```python
from build123d import *

# Parameters (mm, degrees)
BOSS_EXTRUDE1_DEPTH             = 15
H_0_266_DIAMETER_HOLE1_D        = 6.7564
SKETCH5_W                       = 40
SKETCH5_H                       = 16
SKETCH5_W_2                     = 232
SKETCH5_H_2                     = 20.916111238
CUT_EXTRUDE1_DEPTH              = 243.332416321
SKETCH6_W                       = 237.036778435
SKETCH6_H                       = 127.431795429
CUT_EXTRUDE2_DEPTH              = 243.332416321
SKETCH10_W                      = 30
SKETCH10_H                      = 30
BOSS_EXTRUDE3_DEPTH             = 300
SKETCH11_R                      = 6.35
CUT_EXTRUDE4_DEPTH              = 400
SKETCH13_W                      = 600
SKETCH13_H                      = 44.158972604
BOSS_EXTRUDE4_DEPTH             = 3
SKETCH14_W                      = 268.104744415
SKETCH14_H                      = 124.61591485
CUT_EXTRUDE5_DEPTH              = 30
SKETCH15_W                      = 12.7
SKETCH15_H                      = 12.7
CUT_EXTRUDE6_DEPTH              = 385
BOSS_EXTRUDE5_REACH             = 353.137
SKETCH16_R                      = 3.3782
BOSS_EXTRUDE5_DIRECTION_2_REACH = 353.137
CHAMFER1_SIZE                   = 30


with BuildPart() as part:
    # Sketch1 → Boss-Extrude1 (new, symmetric)
    with BuildSketch(Plane.XY):
        with BuildLine():
            Line((-225, 15), (225, 15))
            ThreePointArc((225, 15), (240, 0), (225, -15))
            Line((225, -15), (-225, -15))
            ThreePointArc((-225, -15), (-240, 0), (-225, 15))
        make_face()
    extrude(amount=BOSS_EXTRUDE1_DEPTH, both=True)

    # H (0.266) Diameter Hole1 (through all)
    with Locations(Plane.XY.offset(15)):
        with Locations((-225, 0), (225, 0)):
            Hole(H_0_266_DIAMETER_HOLE1_D / 2)

    # Sketch5 → Cut-Extrude1 (cut, through all)
    with BuildSketch(Plane(origin=(0, 15, 0), x_dir=(1, 0, 0), z_dir=(0, 1, 0))):
        with Locations((-237, 0)):
            Rectangle(SKETCH5_W, SKETCH5_H)
        with Locations((141, 18.458055619)):
            Rectangle(SKETCH5_W_2, SKETCH5_H_2)
        with Locations((141, -18.458055619)):
            Rectangle(SKETCH5_W_2, SKETCH5_H_2)
    extrude(amount=-CUT_EXTRUDE1_DEPTH, mode=Mode.SUBTRACT)

    # Sketch6 → Cut-Extrude2 (cut, through all)
    with BuildSketch(Plane(origin=(0, 15, 0), x_dir=(1, 0, 0), z_dir=(0, 1, 0))):
        with Locations((-293.518389218, -4.674139215)):
            Rectangle(SKETCH6_W, SKETCH6_H)
    extrude(amount=-CUT_EXTRUDE2_DEPTH, mode=Mode.SUBTRACT)

    # Sketch10 → Boss-Extrude3 (add)
    with BuildSketch(Plane.ZY.offset(175)):
        Rectangle(SKETCH10_W, SKETCH10_H)
    extrude(amount=BOSS_EXTRUDE3_DEPTH)

    # Sketch11 → Cut-Extrude4 (cut)
    with BuildSketch(Plane.ZY.offset(475)):
        with Locations((0, 3)):
            Circle(SKETCH11_R)
    extrude(amount=-CUT_EXTRUDE4_DEPTH, mode=Mode.SUBTRACT)

    # Sketch13 → Boss-Extrude4 (add)
    with BuildSketch(Plane(origin=(0, -15, 0), x_dir=(-1, 0, 0), z_dir=(0, -1, 0))):
        with Locations((49.98, 0)):
            Rectangle(SKETCH13_W, SKETCH13_H)
    extrude(amount=BOSS_EXTRUDE4_DEPTH)

    # Sketch14 → Cut-Extrude5 (cut)
    with BuildSketch(Plane(origin=(0, 15, 0), x_dir=(1, 0, 0), z_dir=(0, 1, 0))):
        with Locations((-419.052372208, 3.913950599)):
            Rectangle(SKETCH14_W, SKETCH14_H)
    extrude(amount=-CUT_EXTRUDE5_DEPTH, mode=Mode.SUBTRACT)

    # Sketch15 → Cut-Extrude6 (cut)
    with BuildSketch(Plane.ZY.offset(285)):
        with Locations((0, 3)):
            Rectangle(SKETCH15_W, SKETCH15_H)
    extrude(amount=-CUT_EXTRUDE6_DEPTH, mode=Mode.SUBTRACT)

    # Boss-Extrude5: up to this face of the body (flat: up to its plane)
    boss_extrude5_end = Plane(part.part.faces().sort_by_distance((-130, 0, 15))[0])
    # Sketch16 → Boss-Extrude5 (add, up to the picked face)
    with BuildSketch(Plane.XY, mode=Mode.PRIVATE) as boss_extrude5_sk1:
        with Locations((225, 0)):
            Circle(SKETCH16_R)
    boss_extrude5_tool1 = split(extrude(boss_extrude5_sk1.sketch, amount=BOSS_EXTRUDE5_REACH, mode=Mode.PRIVATE), bisect_by=boss_extrude5_end, keep=Keep.BOTH, mode=Mode.PRIVATE)
    add(boss_extrude5_tool1.solids().sort_by(Axis((225, 0, 0), (0, 0, 1)))[0])

    # Boss-Extrude5 direction 2: up to this face of the body (flat: up to its plane)
    boss_extrude5_direction_2_end = Plane(part.part.faces().sort_by_distance((-130, 0, -15))[0])
    # Sketch16 → Boss-Extrude5 direction 2 (add, up to the picked face)
    with BuildSketch(Plane.XY, mode=Mode.PRIVATE) as boss_extrude5_direction_2_sk1:
        with Locations((225, 0)):
            Circle(SKETCH16_R)
    boss_extrude5_direction_2_tool1 = split(extrude(boss_extrude5_direction_2_sk1.sketch, amount=-BOSS_EXTRUDE5_DIRECTION_2_REACH, mode=Mode.PRIVATE), bisect_by=boss_extrude5_direction_2_end, keep=Keep.BOTH, mode=Mode.PRIVATE)
    add(boss_extrude5_direction_2_tool1.solids().sort_by(Axis((225, 0, 0), (0, 0, -1)))[0])

    # Chamfer1
    chamfer1_edges = [part.edges().sort_by_distance(p)[0] for p in [
        (25, 15, 11.5),
        (25, 15, -11.5),
    ]]
    chamfer(chamfer1_edges, length=CHAMFER1_SIZE - 0.0001)  # a hair under: the kernel refuses the full size


solid = part.part
```
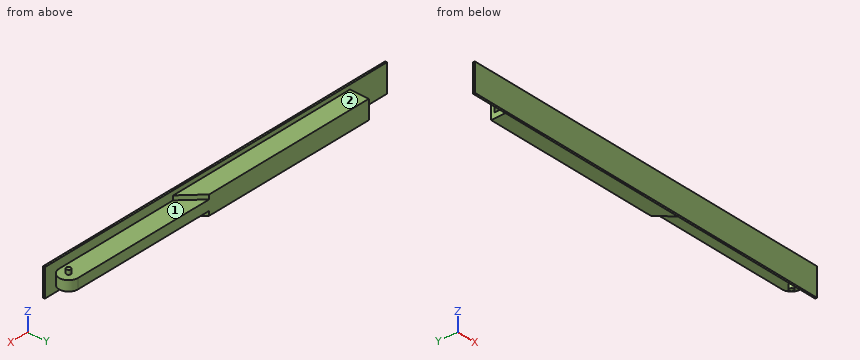
For this review, take the finished solid that the model builds, in its own axes (mm). Face numbers are marked on the shaded views. Coordinates: 2 decimals unless noted, no trailing zeros. Loops run counter-clockwise (first coordinate to the right, second up) from the corner with the lowest first, then second, coordinate; pieces in that order, holes last.
1. Insertion check: P1, Ø3, axis at x = -150, y = 3, coming from the -Z side; P2, Ø5, axis at y = -5.5, z = 2.5, coming from the +X side; P3, Ø3, axis at x = 130, y = 4, coming from the -Z side. Each pin has a flat end and moves straight along its axis. Give the tip position at first contact, or say it passes through.
2. Add section B-B, the plane x = 204. Give the boundary of the cut face in (y, z), then the cut area to 3 significant figures.
3. Mouldability with a two-part tool opening along X and no side actions: class the marked faces 1 and 2 as +X half, -X half, draft (parallel to the pull), parting line (faces both ways), or undercut.
4. Add section A-A, the plane x = -214.5. Give the boundary of the cut face in (y, z), then the cut area to 3 significant figures.
5. For line 1 (Z direction, x = -230, y = 1.5); line 2 (Y direction, x = -316, z = 12.5); line 3 (Z direction, x = 158.5, y = -4.5), list the stretches that pass through material, from the lowest coordinate up.
Result:
1. P1: stops at z = -15
1. P2: stops at x = 239.7
1. P3: stops at z = -8
2. outline: (-18, -22.08) - (-15, -22.08) - (-15, -8) - (15, -8) - (15, 8) - (-15, 8) - (-15, 22.08) - (-18, 22.08) - close
2. area: 612 mm2
3. face 1: undercut
3. face 2: draft
4. outline: (-18, -22.08) - (-15, -22.08) - (-15, -15) - (15, -15) - (15, 15) - (-15, 15) - (-15, 22.08) - (-18, 22.08) - close; hole (-3.35, -6.35) - (9.35, -6.35) - (9.35, 6.35) - (-3.35, 6.35) - close
4. area: 871 mm2
5. line 1: z = -15 to -6.35, 6.35 to 15
5. line 2: y = -18 to -15
5. line 3: z = -8 to 8
